from build123d import *

# Parameters (mm, degrees)
SKETCH_1_R      = 0.4
EXTRUDE_1_DEPTH = 10
SKETCH_2_W      = 60
SKETCH_2_H      = 0.8
EXTRUDE_2_DEPTH = 0.8
FILLET_1_R      = 0.4
SKETCH_3_R      = 0.4
EXTRUDE_3_DEPTH = 5
SKETCH_4_R      = 0.4
EXTRUDE_4_DEPTH = 5
CHAMFER_1_SIZE  = 0.4


with BuildPart() as part:
    # 草图1 → 凸台-拉伸1 (new body)
    with BuildSketch(Plane(origin=(0, 0, 0), x_dir=(1, 0, 0), z_dir=(0, 1, 0))):
        with Locations(Location((0, 0, 0), (0, 0, 270))):
            Circle(SKETCH_1_R)
    extrude(amount=EXTRUDE_1_DEPTH)

    # 草图2 → 凸台-拉伸2 (add)
    with BuildSketch(Plane(origin=(0, 10, 0), x_dir=(1, 0, 0), z_dir=(0, 1, 0))):
        Rectangle(SKETCH_2_W, SKETCH_2_H)
    extrude(amount=EXTRUDE_2_DEPTH)

    # 圆角1
    fillet_1_edges = [part.edges().sort_by_distance(p)[0] for p in [
        (30, 10, 0),
        (30, 10.8, 0),
        (-30, 10, 0),
        (-30, 10.8, 0),
    ]]
    fillet(fillet_1_edges, radius=FILLET_1_R - 0.0001)  # a hair under: the kernel refuses the full size

    # 草图3 → 凸台-拉伸3 (add)
    with BuildSketch(Plane.XY.offset(0.4)):
        with Locations((29.6, 10.4)):
            Circle(SKETCH_3_R)
    extrude(amount=EXTRUDE_3_DEPTH)

    # 草图4 → 凸台-拉伸4 (add)
    with BuildSketch(Plane(origin=(0, 0, -0.4), x_dir=(-1, 0, 0), z_dir=(0, 0, -1))):
        with Locations((29.6, 10.4)):
            Circle(SKETCH_4_R)
    extrude(amount=EXTRUDE_4_DEPTH)

    # 倒角1
    chamfer_1_edges = [part.edges().sort_by_distance(p)[0] for p in [
        (29.2, 10.4, 5.4),
        (-29.2, 10.4, -5.4),
    ]]
    chamfer(chamfer_1_edges, length=CHAMFER_1_SIZE)


solid = part.part
Source: CAD feature listing. Evaluate the final solid. Frame: model axes, mm. Coordinates: 2 decimals unless noted, no trailing zeros. Loops run counter-clockwise (first coordinate to the right, second up) from the corner with the lowest first, then second, coordinate; pieces in that order, holes last. Notation, with made-up numbers: (50, -29) - (95, -29) arc R34 ccw to (95, 4) - close; hole circle Ø4 at (3, 60.25). An arc over 180 degrees is marked (long way). One line per question, with ' | ' between items.
1) First-contact query: P1, Ø0.9, axis at x = 19.5, z = 0, coming from the -Y side; P2, Ø4, axis at y = 6.5, z = 3, coming from the -X side. Flat tips, straight axial feed; report the tip coordinate or a pass-through.
Report:
P1: stops at y = 10 | P2: passes through
2) Section B-B, the plane x = -4.5. Return loops of the section in (y, z), then the cut area to 3 significant figures.
Report:
outline: (10, -0.4) - (10.8, -0.4) - (10.8, 0.4) - (10, 0.4) - close | area: 0.640 mm²
3) Line query: line 1 along X through (y, z) = (1, 0); line 2 along Y through (x, z) = (-27, 0). Output: solid intervals per line, ascending.
Report:
line 1: x = -0.4 to 0.4 | line 2: y = 10 to 10.8
4) Section A-A, the plane z = 3.25. Return loops of the section in (x, y), then the cut area to 3 significant figures.
Report:
outline: circle Ø0.8 at (29.6, 10.4) | area: 0.503 mm²
5) Section C-C, the plane y = 3.5. Return loops of the section in (x, z), then the cut area to 3 significant figures.
Report:
outline: circle Ø0.8 at (0, 0) | area: 0.503 mm²
